Geometry: final body of the model. Coordinates: model frame, mm. Face numbers are marked on the shaded views. A direction names the side the tool comes from. Coordinates: 2 decimals unless noted, no trailing zeros. Loops run counter-clockwise (first coordinate to the right, second up) from the corner with the lowest first, then second, coordinate; pieces in that order, holes last. Notation, with made-up numbers: (-9.5, 38) -> (17.5, 38) arc R19 ccw to (17.5, 50) -> close; hole circle Ø9 at (77.25, 59.5). An arc over 180 degrees is marked (long way). One line per item, written item: value. Start each with the question number.
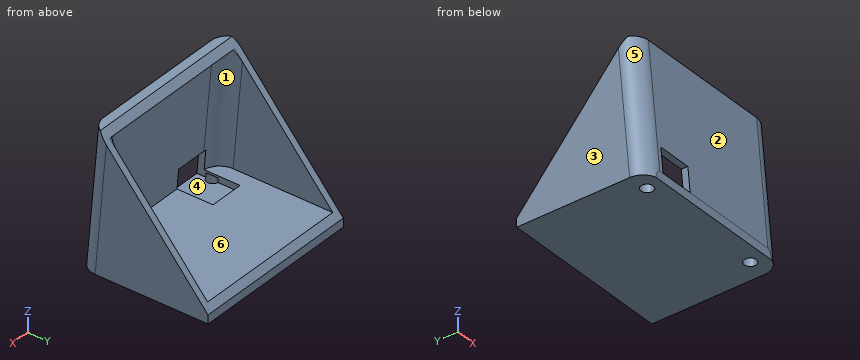
from build123d import *

# Parameters (mm, degrees)
F1_DEPTH     = 40
F2_T         = -1.5
F0_W         = 30
F0_H         = 2
F3_DEPTH     = 40
F4_W         = 8
F4_H         = 6
F5_DEPTH     = 10
F6_R         = 1.4
F7_DEPTH     = 3
F8_T4_DEPTH  = 36.8630372484
F8_T11_DEPTH = 36.8630372484
F8_T17_DEPTH = 36.8630372484
F8_T20_DEPTH = 90


# Not quite as in the source:
# - a fillet or chamfer that OpenCascade refuses, or shapes differently, is made with other operations: its cross-section is extruded or revolved along the edge and cut away or added


with BuildPart() as f1:
    # F0 (on Right) → F1 (new body)
    with BuildSketch(Plane.YZ):
        Polygon((2.6146722824, 29.8858409428), (0, 0), (30, 0), (4.6070616786, 29.7115294573), align=None)
    extrude(amount=F1_DEPTH)

    # F2
    f2_openings = [f1.faces().sort_by_distance(p)[0] for p in [
        (20, 17.303531, 14.855765),
    ]]
    offset(amount=F2_T, openings=f2_openings)

    # F0 (on Right) → F3 (join)
    with BuildSketch(Plane.YZ):
        with Locations((15, -1)):
            Rectangle(F0_W, F0_H)
    extrude(amount=F3_DEPTH)

    # F4 (on Front) → F5 (cut)
    with BuildSketch(Plane.XZ):
        with Locations((9, 3)):
            Rectangle(F4_W, F4_H)
    extrude(amount=-F5_DEPTH, mode=Mode.SUBTRACT)

    # F6 (on face) → F7 (cut)
    with BuildSketch(Plane(origin=(0, 0, -2), x_dir=(1, 0, 0), z_dir=(0, 0, -1))):
        with Locations((4.75, -3.5)):
            Circle(F6_R)
        with Locations((35.25, -3.5)):
            Circle(F6_R)
    extrude(amount=-F7_DEPTH, mode=Mode.SUBTRACT)

    # F8: fillet of radius 4 on 4 edges, made by hand


with BuildPart() as f8_tool2:
    # F8_s3 → F8_t4 (new body)
    with BuildSketch(Plane(origin=(0, -0.728886723, -8.3312133668), x_dir=(1, 0, 0), z_dir=(0, 0.0871557427, 0.9961946981))):
        with BuildLine():
            ThreePointArc((5.5, 1.5), (2.6715728753, 2.6715728753), (1.5, 5.5))
            Line((1.5, 5.5), (1.5, 1.5))
            Line((1.5, 1.5), (5.5, 1.5))
        make_face()
    extrude(amount=F8_T4_DEPTH)

    split(bisect_by=Plane.YZ.offset(5), keep=Keep.BOTTOM)

    split(bisect_by=Plane(origin=(0, 17.3367768884, 14.8168645055), x_dir=(1, 0, 0), z_dir=(0, -0.7601924513, -0.6496979583)), keep=Keep.TOP)

    split(bisect_by=Plane.XY.offset(1.5), keep=Keep.TOP)


with BuildPart() as f1_1:
    add(f1.part)

    # F8_t1: union F8_tool2
    add(f8_tool2.part)


with BuildPart() as f8_tool9:
    # F8_s10 → F8_t11 (new body)
    with BuildSketch(Plane(origin=(0, -0.728886723, -8.3312133668), x_dir=(1, 0, 0), z_dir=(0, 0.0871557427, 0.9961946981))):
        with BuildLine():
            ThreePointArc((5.5, 1.5), (2.6715728753, 2.6715728753), (1.5, 5.5))
            Line((1.5, 5.5), (1.5, 1.5))
            Line((1.5, 1.5), (5.5, 1.5))
        make_face()
    extrude(amount=F8_T11_DEPTH)

    split(bisect_by=Plane.XY.offset(6), keep=Keep.TOP)

    split(bisect_by=Plane(origin=(0, 17.3367768884, 14.8168645055), x_dir=(1, 0, 0), z_dir=(0, -0.7601924513, -0.6496979583)), keep=Keep.TOP)


with BuildPart() as f1_2:
    add(f1_1.part)

    # F8_t8: union F8_tool9
    add(f8_tool9.part)


with BuildPart() as f8_tool15:
    # F8_s16 → F8_t17 (new body)
    with BuildSketch(Plane(origin=(0, -0.728886723, -8.3312133668), x_dir=(1, 0, 0), z_dir=(0, 0.0871557427, 0.9961946981))):
        with BuildLine():
            ThreePointArc((34.5, 1.5), (37.3284271247, 2.6715728753), (38.5, 5.5))
            Line((38.5, 5.5), (38.5, 1.5))
            Line((38.5, 1.5), (34.5, 1.5))
        make_face()
    extrude(amount=F8_T17_DEPTH)

    split(bisect_by=Plane(origin=(0, 17.3367768884, 14.8168645055), x_dir=(1, 0, 0), z_dir=(0, -0.7601924513, -0.6496979583)), keep=Keep.TOP)

    split(bisect_by=Plane.XY.offset(1.5), keep=Keep.TOP)


with BuildPart() as f1_3:
    add(f1_2.part)

    # F8_t14: union F8_tool15
    add(f8_tool15.part)

    # F8_s21 → F8_t20 (cut)
    with BuildSketch(Plane(origin=(0, 3.4862297099, 39.8477879237), x_dir=(1, 0, 0), z_dir=(0, -0.0871557427, -0.9961946981))):
        with BuildLine():
            ThreePointArc((4, 0), (1.1715728753, -1.1715728753), (0, -4))
            Line((0, -4), (0, 0))
            Line((0, 0), (4, 0))
        make_face()
        with BuildLine():
            ThreePointArc((36, 0), (38.8284271247, -1.1715728753), (40, -4))
            Line((40, -4), (40, 0))
            Line((40, 0), (36, 0))
        make_face()
    extrude(amount=F8_T20_DEPTH, mode=Mode.SUBTRACT)


solid = f1_3.part
1. Set-up query: the marked faces 5 and 6. Return all of +Z, -Z, +X, -X, +Y, -Y with unobstructed straight access to the full face (end or side cutting, diameter ignored); none if empty.
2. Section D-D on y = 17. Return the cut outline in (x, z), plus the area to 3 significant figures.
3. Draft query along Z for the marked faces 1, 2, 3 and 4. Return one class per face: released by +Z, released by -Z, zero draft, split by the parting line, or undercut.
4. Line query: L1, parallel to X at y = 16.5, z = 6.5; L2, parallel to X at y = 3.5, z = -1.1; L3, parallel to X at y = 3.5, z = 0.1. Output: solid intervals per line, ascending. Write a range as [from, to].
5. Section A-A on x = 31.5. Return the cut outline in (y, z), plus the area to 3 significant figures.
6. Section C-C on y = 11.75. Return the cut outline in (x, z).
7. Section B-B on x = 7. Return the cut outline in (y, z), plus the area to 3 significant figures.
8. Pin query (flat end, axial travel): pin 1 Ø3 at (x, y) = (24, 25.5) entering from +Z; pin 2 Ø3 at (y, z) = (4.5, 24.5) entering from -X; pin 3 Ø4 at (x, z) = (36, 9) entering from -Y. Return the tip coordinate at first contact, or that it passes through.
Checks:
1. face 5: +Z, -X, -Y
1. face 6: +Y
2. outline: (0, -2) -> (40, -2) -> (40, 15.21) -> (38.5, 15.21) -> (38.5, 1.5) -> (1.5, 1.5) -> (1.5, 15.21) -> (0, 15.21) -> close
2. area: 181 mm²
3. face 1: undercut
3. face 2: released by +Z
3. face 3: zero draft
3. face 4: undercut
4. L1: [0, 1.5], [38.5, 40]
4. L2: [0.02, 3.35], [6.15, 33.85], [36.65, 39.98]
4. L3: [0.03, 3.35], [13, 33.85], [36.65, 39.97]
5. outline: (0, -2) -> (30, -2) -> (30, 0) -> (28.72, 1.5) -> (1.64, 1.5) -> (3.98, 28.26) -> (6, 28.08) -> (4.61, 29.71) -> (2.61, 29.89) -> (0, 0) -> close
5. area: 148 mm²
6. outline: (0, -2) -> (40, -2) -> (40, 21.35) -> (38.5, 21.35) -> (38.5, 1.5) -> (1.5, 1.5) -> (1.5, 21.35) -> (0, 21.35) -> close
7. outline: (0, -2) -> (30, -2) -> (30, 0) -> (28.72, 1.5) -> (10, 1.5) -> (10, 0) -> (0, 0) -> close; (0.52, 6) -> (2.03, 6) -> (3.98, 28.26) -> (6, 28.08) -> (4.61, 29.71) -> (2.61, 29.89) -> close
7. area: 127 mm²
8. pin 1: z = 1.5
8. pin 2: x = 0
8. pin 3: y = 0.61
